Autodesk Inventor part; units mm, degrees
ref_plane "YZ Plane" through (0, 0, 0) normal (1, 0, 0) x (0, 1, 0)
ref_plane "XZ Plane" through (0, 0, 0) normal (0, 1, 0) x (-1, 0, 0)
ref_plane "XY Plane" through (0, 0, 0) normal (0, 0, 1) x (1, 0, 0)
sketch "Sketch1" plane through (0, 0, 0) normal (0, 0, 1) x (1, 0, 0)
  line L0 (0, 25.4) -> (-25.4, 25.4)
  line L1 (-25.4, 25.4) -> (-47.397, 63.5)
  line L2 (-47.397, 63.5) -> (-66.447, 63.5)
  line L3 (-66.447, 63.5) -> (-66.447, 38.1)
  line L4 (-66.447, 38.1) -> (-79.147, 38.1)
  line L5 (0, -12.7) -> (0, 76.2)
  line L6 (-110.8059, 0) -> (110.8059, 0)
  line L7 (0, 25.4) -> (25.4, 25.4)
  line L8 (25.4, 25.4) -> (47.397, 63.5)
  line L9 (47.397, 63.5) -> (66.447, 63.5)
  line L10 (66.447, 63.5) -> (66.447, 38.1)
  line L11 (66.447, 38.1) -> (79.147, 38.1)
  line L12 (79.147, 38.1) -> (79.147, 0)
  line L13 (-79.147, 38.1) -> (-79.147, 0)
  line L14 (-79.147, 0) -> (79.147, 0)
  point P0 (0, 0)
  dimension "d3" = 19.05
  dimension "d13" = 60
  dimension "d14" = 12.7
  dimension "d15" = 127
  dimension "d16" = 76.2
  dimension "d17" = 50.8
  dimension "d18" = 50.8
revolve "Revolution1" add sketch "Sketch1" angle 360 about axis through (-79.147, 0, 0) along (1, 0, 0)
properties part number "Ch3 Part 3"
Geometry: final body of the model. Coordinates: model frame, mm. A direction names the side the tool comes from. Coordinates: 2 decimals unless noted, no trailing zeros. Order: outer loops, then holes, each group sorted by start corner. A loop starts at its lowest first (then second) coordinate and runs counter-clockwise, first axis right, second up.
1) Section C-C (x = -59.5). Return loops of the section in (y, z).
Result sheet:
outline: circle Ø127 at (0, 0)
2) Section A-A (z = 0). Return loops of the section in (x, y), then the cut area to 3 significant figures.
Result sheet:
outline: (-79.15, -38.1) - (-66.45, -38.1) - (-66.45, -63.5) - (-47.4, -63.5) - (-25.4, -25.4) - (25.4, -25.4) - (47.4, -63.5) - (66.45, -63.5) - (66.45, -38.1) - (79.15, -38.1) - (79.15, 38.1) - (66.45, 38.1) - (66.45, 63.5) - (47.4, 63.5) - (25.4, 25.4) - (-25.4, 25.4) - (-47.4, 63.5) - (-66.45, 63.5) - (-66.45, 38.1) - (-79.15, 38.1) - close
area: 13,300 mm2
3) Set-up query: faces 1 (the cylindrical face through (72.886, -30.235, -23.183)), 2 (the flat face through (-79.147, -1, 1)), 3 (the conical face through (26.776, 12.82, -24.649)). Return all of +Z, -Z, +X, -X, +Y, -Y with unobstructed straight access to the full face (end or side cutting, diameter ignored); none if empty.
Result sheet:
face 1: +X
face 2: +Z, -Z, -X, +Y, -Y
face 3: none
4) Section D-D (x = 14). Return loops of the section in (y, z).
Result sheet:
outline: circle Ø50.8 at (0, 0)
5) First-contact query: P1, Ø10, axis at x = -25.5, y = -40, coming from the +Z side; P2, Ø1, axis at x = -31, y = -11, coming from the +Z side; P3, Ø8, axis at x = -35.5, y = 23, coming from the -Z side; P4, Ø3, axis at y = 44, z = -5.5, coming from the -X side. Flat tips, straight axial feed; report the tip coordinate or a pass-through.
Result sheet:
P1: passes through
P2: stops at z = 34.26
P3: stops at z = -44.46
P4: stops at x = -66.45
6) Draft query along X for faces 4 (the cylindrical face through (-72.886, -30.235, 23.183)), 5 (the cylindrical face through (-0.356, -5.506, 24.796)), 6 (the flat face through (-66.447, 27.3, -27.3)), 7 (the flat face through (66.447, 27.3, -27.3)). Return one class per face: released by +X, released by -X, zero draft, split by the parting line, or undercut.
Result sheet:
face 4: zero draft
face 5: undercut
face 6: released by -X
face 7: released by +X
7) Ray query, probe 1 along X at (y, z) = (26.5, 1); probe 2 along X at (y, z) = (-21.5, -58); probe 3 along Z at (x, y) = (-23.5, -4.5). Return the intervals inside material, ascending.
Result sheet:
probe 1: x = -79.15 to -26.05, 26.05 to 79.15
probe 2: x = -66.45 to -46.45, 46.45 to 66.45
probe 3: z = -25 to 25
